Design review of the part built by this model. Coordinates are the model's own, in mm. Give positions to 0.01 mm unless a question says otherwise; leave off trailing zeros. Loops run counter-clockwise (first coordinate to the right, second up) from the corner with the lowest first, then second, coordinate; pieces in that order, holes last. Notation, with made-up numbers: (11, -15) - (68, -15) arc R27 cw to (68, 5) - close; hole circle Ø8 at (46.25, 77.25). An arc over 180 degrees is marked (long way). Write each question's results on one line, items separated by ' | '.
from build123d import *

# Parameters (mm, degrees)
SKETCH1_R           = 2.54
SKETCH1_R_2         = 14.2875
BOSS_EXTRUDE1_DEPTH = 3.175


with BuildPart() as part:
    # Sketch1 → Boss-Extrude1 (new body)
    with BuildSketch(Plane.XY):
        with BuildLine():
            Line((0, 0), (0, 50.8))
            Line((0, 50.8), (50.8, 50.534405745))
            Line((50.8, 50.534405745), (76.2, 50.534405745))
            ThreePointArc((76.2, 50.534405745), (101.467202873, 25.267202873), (76.2, 0))
            Line((76.2, 0), (0, 0))
        make_face()
        with Locations((12.7, 37.900630736)):
            Circle(SKETCH1_R, mode=Mode.SUBTRACT)
        with Locations((25.4, 37.900630736)):
            Circle(SKETCH1_R, mode=Mode.SUBTRACT)
        with Locations((38.1, 37.900630736)):
            Circle(SKETCH1_R, mode=Mode.SUBTRACT)
        with Locations((25.4, 25.200630736)):
            Circle(SKETCH1_R, mode=Mode.SUBTRACT)
        with Locations((38.1, 25.200630736)):
            Circle(SKETCH1_R, mode=Mode.SUBTRACT)
        with Locations((25.4, 12.500630736)):
            Circle(SKETCH1_R, mode=Mode.SUBTRACT)
        with Locations((38.1, 12.500630736)):
            Circle(SKETCH1_R, mode=Mode.SUBTRACT)
        with Locations((12.7, 25.200630736)):
            Circle(SKETCH1_R, mode=Mode.SUBTRACT)
        with Locations((12.7, 12.500630736)):
            Circle(SKETCH1_R, mode=Mode.SUBTRACT)
        with Locations((76.2, 25.267202873)):
            Circle(SKETCH1_R_2, mode=Mode.SUBTRACT)
    extrude(amount=BOSS_EXTRUDE1_DEPTH)


solid = part.part
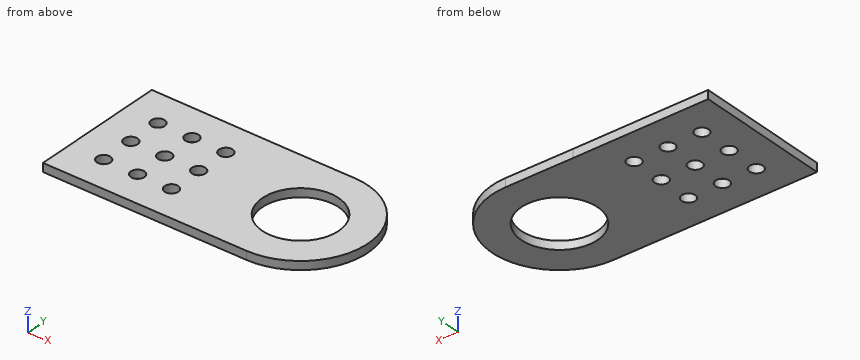
(1) Take a section at D-D on z = 0.7. Count the separate pieces of the cut face and the enclosed holes in it, plus the area to 3 significant figures.
Answers below:
separate pieces: 1 | enclosed holes: 10 | area: 4,040 mm2
(2) Wall thickness on line 1 along Y through (x, z) = (38.1, 0.9); line 2 along X through (y, z) = (38.5, 2.95); line 3 along X through (y, z) = (24.5, 0.2): over which ranges is each line inside the solid? List them lowest first. Write a range as from..to.
Answers below:
line 1: 0..9.96, 15.04..22.66, 27.74..35.36, 40.44..50.6 | line 2: 0..10.23, 15.17..22.93, 27.87..35.63, 40.57..70.81, 81.59..97.72 | line 3: 0..10.26, 15.14..22.96, 27.84..35.66, 40.54..61.93, 90.47..101.46
(3) Take a section at C-C on x = 25.4. Give the boundary of the cut face in (y, z) (3 decimals).
Answers below:
outline: (0, 0) - (9.961, 0) - (9.961, 3.175) - (0, 3.175) - close; (15.041, 0) - (22.661, 0) - (22.661, 3.175) - (15.041, 3.175) - close; (27.741, 0) - (35.361, 0) - (35.361, 3.175) - (27.741, 3.175) - close; (40.441, 0) - (50.667, 0) - (50.667, 3.175) - (40.441, 3.175) - close
(4) Take a section at A-A on x = 81. Give the boundary of the cut face in (y, z) (3 decimals), plus the area to 3 significant figures.
Answers below:
outline: (0.46, 0) - (11.81, 0) - (11.81, 3.175) - (0.46, 3.175) - close; (38.724, 0) - (50.074, 0) - (50.074, 3.175) - (38.724, 3.175) - close | area: 72.1 mm2
(5) Take a section at B-B on y = 33.5. Give the boundary of the cut face in (x, z) (3 decimals), plus the area to 3 significant figures.
Answers below:
outline: (0, 0) - (64.523, 0) - (64.523, 3.175) - (0, 3.175) - close; (87.877, 0) - (100.088, 0) - (100.088, 3.175) - (87.877, 3.175) - close | area: 244 mm2
(6) Insertion check: P1, Ø4, axis at x = 25.4, y = 25.2, coming from the -Z side; P2, Ø1.5, axis at x = 57.5, z = 1.5, coming from the +Y side. Each pin has a flat end and moves straight along its axis. Give the tip position at first contact, or say it passes through.
Answers below:
P1: through | P2: y = 50.53
